Answer from the drawing. Dimensions are ordinates in mm from the lowest x, y and z of the part. A direction names the side the tool comes from. Give positions to 0.01 mm unless a question says otherwise; leave off trailing zeros. Loops run counter-clockwise (first coordinate to the right, second up) from the corner with the lowest first, then second, coordinate; pieces in that order, holes last. Notation, with made-up numbers: (2, 0) - (24, 0) arc R17 cw to (24, 33) - close; hole circle Ø4 at (15, 28). An arc over 180 degrees is marked (long way). Put each result on its own line as item: value. Start each with the question number.
1. Consider L1, parallel to Y at x = 0.35, z = 3.5; L2, parallel to Z at x = 0.6, y = 25; L3, parallel to Y at x = 16, z = 28.5. Determine where each line is inside the solid, lowest interval first. Write a range as from..to.
2. A cutting plane is placed at A-A, the plane y = 17. Determine the outline of the cut face in (x, z).
3. A cutting plane is placed at B-B, the plane z = 3.5. Determine the outline of the cut face in (x, y), plus the area to 3 significant figures.
4. A cutting plane is placed at C-C, the plane y = 9. Determine the outline of the cut face in (x, z), plus the area to 3 significant figures.
5. Given pin 1 Ø12 at (x, z) = (29, 30.5) entering from +Y; pin 2 Ø0.8 at (y, z) = (0.5, 70.5) entering from +X; pin 3 Ø10 at (x, y) = (36, 13) entering from -Z; pin 4 Ø0.5 at (y, z) = (0.5, 46.5) entering from -X, each flat-ended and moving along its own axis, determine where each tip first touches the part or whether it passes through.
6. A cutting plane is placed at D-D, the plane x = 6. Determine the outline of the cut face in (y, z), plus the area to 3 significant figures.
7. For the marked faces 1, 2 and 3, determine the directions among +Z, -Z, +X, -X, +Y, -Y from which every point of the face is accessible in a straight line to the end or side of a thin tool.
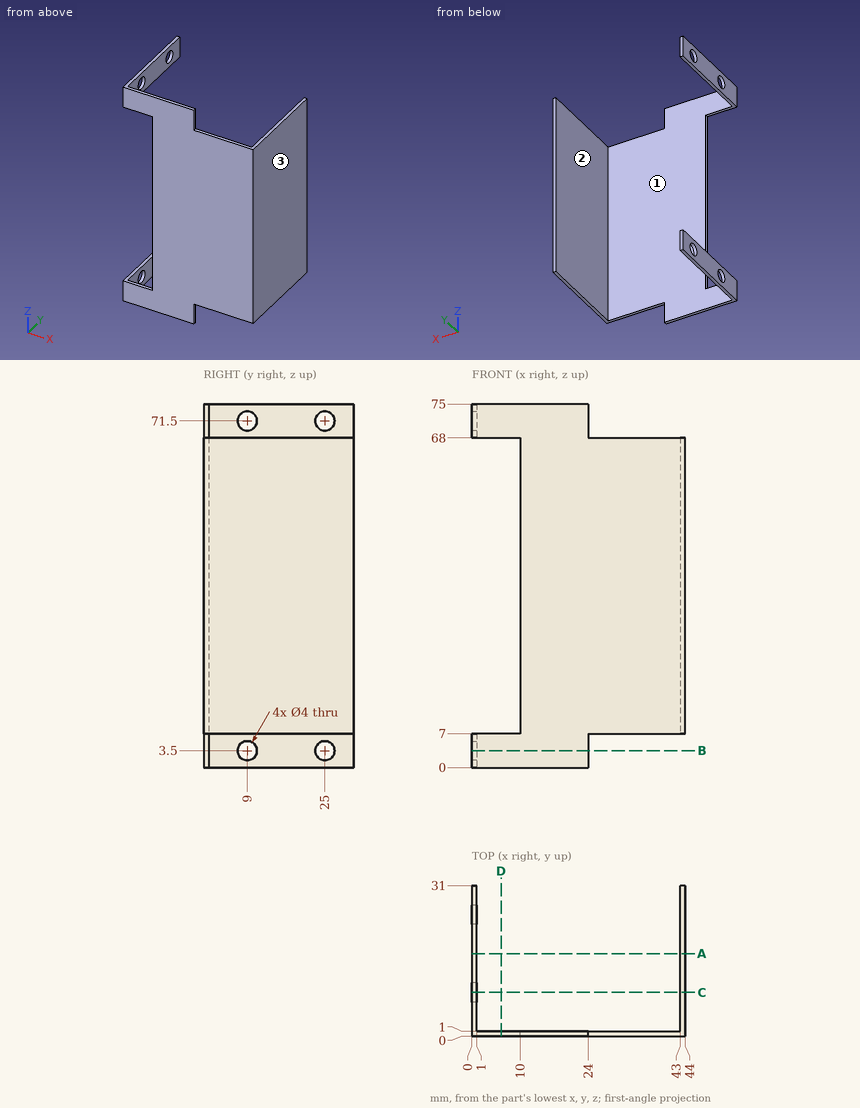
Return value:
1. L1: y = 0..7, 11..23, 27..31
1. L2: z = 0..1.5, 5.5..7, 68..69.5, 73.5..75
1. L3: y = 0..1
2. outline: (0, 0) - (1, 0) - (1, 7) - (0, 7) - close; (0, 68) - (1, 68) - (1, 75) - (0, 75) - close; (43, 7) - (44, 7) - (44, 68) - (43, 68) - close
3. outline: (0, 0) - (24, 0) - (24, 1) - (1, 1) - (1, 7) - (0, 7) - close; (0, 11) - (1, 11) - (1, 23) - (0, 23) - close; (0, 27) - (1, 27) - (1, 31) - (0, 31) - close
3. area: 46.0 mm2
4. outline: (0, 0) - (1, 0) - (1, 1.5) - (0, 1.5) - close; (0, 5.5) - (1, 5.5) - (1, 7) - (0, 7) - close; (0, 68) - (1, 68) - (1, 69.5) - (0, 69.5) - close; (0, 73.5) - (1, 73.5) - (1, 75) - (0, 75) - close; (43, 7) - (44, 7) - (44, 68) - (43, 68) - close
4. area: 67.0 mm2
5. pin 1: stops at y = 1
5. pin 2: stops at x = 24
5. pin 3: passes through
5. pin 4: stops at x = 10
6. outline: (0, 0) - (1, 0) - (1, 7) - (0, 7) - close; (0, 68) - (1, 68) - (1, 75) - (0, 75) - close
6. area: 14.0 mm2
7. face 1: +Z, -Z, +Y
7. face 2: +Z, -Z, -X, +Y
7. face 3: +Z, -Z, +X, +Y, -Y
